Design review of the part built by this model. Coordinates are the model's own, in mm. Give positions to 0.01 mm unless a question says otherwise; leave off trailing zeros. Write each loop counter-clockwise with the first axis right and the second up, starting at its lowest first coordinate (ties: lowest second). Pieces come first, ordered by that corner, then holes. Notation, with made-up numbers: M 4.5,13.25 L 19.5,13.25 A22 cw 19.5,31.25 Z; hole C 17.5,0.25 d3. An arc over 180 degrees is marked long. Answer in a Markdown table with one row per item.
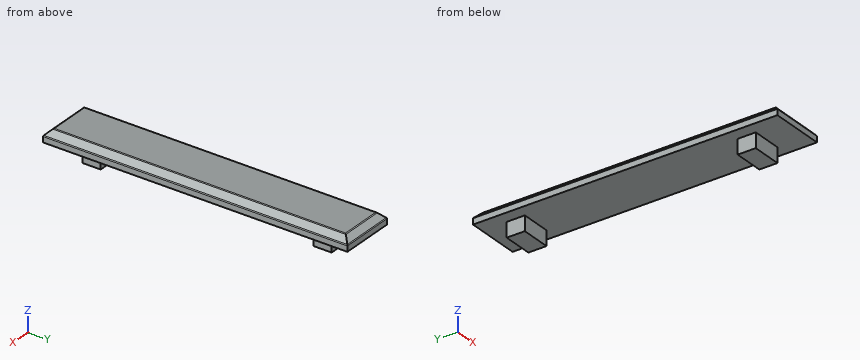
Autodesk Fusion 360 part; units mm, degrees
sketch "Sketch1" plane through (0, 0, 0) normal (0, 0, 1) x (1, 0, 0)
  line L0 (9, 50) -> (-9, 50)
  line L1 (-9, 50) -> (-9, -50)
  line L2 (-9, -50) -> (9, -50)
  line L3 (9, -50) -> (9, 50)
  line L4 (9, 50) -> (-9, -50) construction
  line L5 (-9, 50) -> (9, -50) construction
  line L6 (-4.925, 41.8706) -> (4.925, 41.8706)
  line L7 (4.925, 41.8706) -> (4.925, 35.9206)
  line L8 (4.925, 35.9206) -> (-4.925, 35.9206)
  line L9 (-4.925, 35.9206) -> (-4.925, 41.8706)
  line L10 (-4.925, 41.8706) -> (4.925, 35.9206) construction
  line L11 (4.925, 41.8706) -> (-4.925, 35.9206) construction
  line L12 (4.925, -33.9994) -> (-4.925, -33.9994)
  line L13 (-4.925, -33.9994) -> (-4.925, -39.9494)
  line L14 (-4.925, -39.9494) -> (4.925, -39.9494)
  line L15 (4.925, -39.9494) -> (4.925, -33.9994)
  line L16 (4.925, -33.9994) -> (-4.925, -39.9494) construction
  line L17 (-4.925, -33.9994) -> (4.925, -39.9494) construction
  point P0 (0, 38.8956)
  point P1 (0, -36.9744)
  dimension "d1" = 18
  dimension "d2" = 100
  dimension "d3" = 5.95
  dimension "d4" = 9.85
  dimension "d5" = 5.95
  dimension "d9" = 4.925
  dimension "d10" = 33.9994
  dimension "d11" = 69.92
extrude "Extrude1" add sketch "Sketch1" against normal blind 4.85 contours L6 L7 L8 L9 | L12 L13 L14 L15 makes body 1 at (-1.6417, 37.9039, 0) makes body 2 at (1.6417, -35.9827, 0)
sketch "Sketch2" plane through (0, 0, 0) normal (0, 0, 1) x (1, 0, 0)
  line L0 (9, 50) -> (-9, 50)
  line L1 (-9, 50) -> (-9, -50)
  line L2 (-9, -50) -> (9, -50)
  line L3 (9, -50) -> (9, 50)
  line L4 (9, 50) -> (-9, -50) construction
  line L5 (-9, 50) -> (9, -50) construction
  dimension "d14" = 18
  dimension "d15" = 100
extrude "Extrude2" add sketch "Sketch2" along normal blind 4 bodies 1 2
chamfer "Chamfer1" distance 2 angle 45 1 faces at (-3, -16.6667, 4) on bodies 1
fillet "Fillet1" radius 0.5 8 edges at (-7, 0, 4) (0, -48, 4) (7, 0, 4) (0, 48, 4) (-9, 0, 2) (0, -50, 2) (0, 50, 2) (9, 0, 2) on bodies 1
1) Add section B-B (y = 40.5). Write out the cut boundary in (x, z) (3 decimals).
Geometry says:
| item | result |
|---|---|
| outline | M -9,0 L -4.925,0 L -4.925,-4.85 L 4.925,-4.85 L 4.925,0 L 9,0 L 9,1.793 A0.5 ccw 8.854,2.146 L 7.146,3.854 A0.5 ccw 6.793,4 L -6.793,4 A0.5 ccw -7.146,3.854 L -8.854,2.146 A0.5 ccw -9,1.793 Z |
2) Add section C-C (x = -3.5). Write out the cut boundary in (y, z).
Geometry says:
| item | result |
|---|---|
| outline | M -50,0 L -39.95,0 L -39.95,-4.85 L -34,-4.85 L -34,0 L 35.92,0 L 35.92,-4.85 L 41.87,-4.85 L 41.87,0 L 50,0 L 50,1.79 A0.5 ccw 49.85,2.15 L 48.15,3.85 A0.5 ccw 47.79,4 L -47.79,4 A0.5 ccw -48.15,3.85 L -49.85,2.15 A0.5 ccw -50,1.79 Z |
3) To check wall thickness, follow probe 1 along Y at (x, z) = (3.75, -1); probe 2 along X at (y, z) = (40.5, -3.25) (3 decimals); probe 3 along Z at (x, y) = (-2.75, 4). State the ranges of each line that lie inside material, in increasing order. Write a range as [from, to].
Geometry says:
| item | result |
|---|---|
| probe 1 | [-39.95, -34], [35.92, 41.87] |
| probe 2 | [-4.925, 4.925] |
| probe 3 | [0, 4] |
4) Add section D-D (y = 2.5). Write out the cut boundary in (x, z), and give its area (3 significant figures).
Geometry says:
| item | result |
|---|---|
| outline | M -9,0 L 9,0 L 9,1.79 A0.5 ccw 8.85,2.15 L 7.15,3.85 A0.5 ccw 6.79,4 L -6.79,4 A0.5 ccw -7.15,3.85 L -8.85,2.15 A0.5 ccw -9,1.79 Z |
| area | 68.0 mm^2 |
5) Insertion check: P1, Ø2.5, axis at x = 0, z = -2.5, coming from the -Y side; P2, Ø1.5, axis at y = -36, z = -2.5, coming from the +X side (3 decimals); P3, Ø1.5, axis at x = 0, z = -3.5, coming from the +Y side. Each pin has a flat end and moves straight along its axis. Give the tip position at first contact, or say it passes through.
Geometry says:
| item | result |
|---|---|
| P1 | y = -39.95 |
| P2 | x = 4.925 |
| P3 | y = 41.87 |
6) Add section A-A (z = -1). Write out the cut boundary in (x, y) (3 decimals).
Geometry says:
| item | result |
|---|---|
| outline | M -4.925,-39.949 L 4.925,-39.949 L 4.925,-33.999 L -4.925,-33.999 Z; M -4.925,35.921 L 4.925,35.921 L 4.925,41.871 L -4.925,41.871 Z |
